```python
from build123d import *

# Parameters (mm, degrees)
F1_DEPTH = 25.4
F3_DEPTH = 25.4


with BuildPart() as f1:
    # F0 (on Right) → F1 (new body)
    with BuildSketch(Plane.YZ):
        Polygon((0, 25.4), (0, 0), (25.4, 0), (25.4, 25.4), (19.05, 25.4), (19.05, 12.7), (6.35, 12.7), (6.35, 25.4), align=None)
    extrude(amount=F1_DEPTH)

    # F2 (on face) → F3 (cut)
    with BuildSketch(Plane.XZ):
        Polygon((25.4, 25.4), (19.05, 25.4), (25.4, 0), align=None)
    extrude(amount=-F3_DEPTH, mode=Mode.SUBTRACT)


solid = f1.part
```
The listing builds one solid part. Answer for the finished solid, in the listing's coordinates (mm). A direction names the side the tool comes from. Round coordinates to 2 decimals unless told otherwise and drop trailing zeros. Loops run counter-clockwise (first coordinate to the right, second up) from the corner with the lowest first, then second, coordinate; pieces in that order, holes last.
Q1. Which of the six approach directions +Z, -Z, +X, -X, +Y, -Y give full straight-line access (tool end or side, diameter ignored) to faces 1 (the face through (11, 6.35, 19)), 2 (the face through (9, 22, 25.4))?
Q2. Find the intervals of material crossed by line 1 (Y direction, x = 19.5, z = 15); line 2 (Z direction, x = 3.5, y = 14.5); line 3 (X direction, y = 23.5, z = 10), in increasing order.
Q3. Section B-B, the plane z = 21.5 is taken. Determine the outline of the cut face in (x, y) (3 decimals), then the cut area to 3 significant figures.
Q4. Section A-A, the plane x = 8.5 is taken. Determine the outline of the cut face in (y, z), then the cut area to 3 significant figures.
Q5. For a pull along Y with two mould halves and no side action, classify faces 3 (the face through (11, 19.05, 19)), 4 (the face through (22.886, 12.522, 10.056)), 5 (the face through (11, 13, 12.7)), 6 (the face through (10, 25.4, 13)) as released by +Y, released by -Y, zero draft, split by the parting line, or undercut.
Q6. Section D-D, the plane z = 13.75 is taken. Determine the outline of the cut face in (x, y), then the cut area to 3 significant figures.
Q7. Given pin 1 Ø1.5 at (x, y) = (5, 17.5) entering from +Z; pin 2 Ø6 at (x, z) = (16.5, 6) entering from -Y; pin 3 Ø5 at (y, z) = (8.5, 3.5) entering from +X; pin 4 Ø8 at (y, z) = (12.5, 16) entering from +X, each flat-ended and moving along its own axis, determine where each tip first touches the part or whether it passes through.
Q8. Section C-C, the plane y = 14.5 is taken. Determine the outline of the cut face in (x, z) (3 decimals).
Completed:
1. face 1: +Z, +X, -X
1. face 2: +Z, +X, -X, +Y, -Y
2. line 1: y = 0 to 6.35, 19.05 to 25.4
2. line 2: z = 0 to 12.7
2. line 3: x = 0 to 22.9
3. outline: (0, 0) - (20.025, 0) - (20.025, 6.35) - (0, 6.35) - close; (0, 19.05) - (20.025, 19.05) - (20.025, 25.4) - (0, 25.4) - close
3. area: 254 mm2
4. outline: (0, 0) - (25.4, 0) - (25.4, 25.4) - (19.05, 25.4) - (19.05, 12.7) - (6.35, 12.7) - (6.35, 25.4) - (0, 25.4) - close
4. area: 484 mm2
5. face 3: undercut
5. face 4: zero draft
5. face 5: undercut
5. face 6: released by +Y
6. outline: (0, 0) - (21.96, 0) - (21.96, 6.35) - (0, 6.35) - close; (0, 19.05) - (21.96, 19.05) - (21.96, 25.4) - (0, 25.4) - close
6. area: 279 mm2
7. pin 1: stops at z = 12.7
7. pin 2: stops at y = 0
7. pin 3: stops at x = 25.15
7. pin 4: stops at x = 22.4
8. outline: (0, 0) - (25.4, 0) - (22.225, 12.7) - (0, 12.7) - close
